Check sheet for the modelled part. Datum: model origin and axes. Units: mm. A direction names the side the tool comes from. Give positions to 0.01 mm unless a question says otherwise; leave off trailing zeros. Loops run counter-clockwise (first coordinate to the right, second up) from the corner with the lowest first, then second, coordinate; pieces in that order, holes last. Notation, with made-up numbers: M 5,28.5 L 58,28.5 A27 ccw 58,44.5 Z; hole C 4,82.25 d11. An arc over 180 degrees is marked long. Write each question's results on one line, items separated by ' | '. Start each with the question number.
1. Sectioned sample at C-C on z = -40.5. Record the cut outline in (x, y), and give its area (3 significant figures).
2. Sectioned sample at A-A on y = 0.25. Record the cut outline in (x, z), and give its area (3 significant figures).
3. Material ranges on line 1 along Z through (x, y) = (0.5, 9.75); line 2 along X through (y, z) = (-0.25, -38.5); line 3 along Y through (x, z) = (12, -32), recorded low to high.
4. Tool access check on faces 1 (the flat face through (0, -3.492, -30)), 2 (the flat face through (-17.78, 0, -30)), 3 (the flat face through (17.78, 0, -30)), 4 (the flat face through (0, 3.492, -30)). Record the directions out of +Z, -Z, +X, -X, +Y, -Y that give a thin tool (end or side, any length) a straight path to the whole face; none if there is none.
5. Sectioned sample at D-D on y = -9.25. Record the cut outline in (x, z), and give its area (3 significant figures).
6. Sectioned sample at B-B on x = 15. Record the cut outline in (y, z), and give its area (3 significant figures).
7. Go/stop test with flat-tipped pins: pin 1 (5 mm diameter, centred on x = -8.5, z = -36, fed in from -Y); pin 2 (2 mm diameter, centred on x = -26, y = 11, fed in from -Z); pin 3 (1 mm diameter, centred on x = 3, z = -37, fed in from +Y). Record where each tip stops, or that it passes through.
```python
from build123d import *

# Parameters (mm, degrees)
SKETCH1_W           = 70.0024
SKETCH1_H           = 22.9616
BOSS_EXTRUDE1_DEPTH = 14.9098
SKETCH2_W           = 35.56
SKETCH2_H           = 6.985
BOSS_EXTRUDE2_DEPTH = 38.1


with BuildPart() as part:
    # Sketch1 → Boss-Extrude1 (new, symmetric)
    with BuildSketch(Plane(origin=(0, 0, 0), x_dir=(1, 0, 0), z_dir=(0, 1, 0))):
        Rectangle(SKETCH1_W, SKETCH1_H)
    extrude(amount=BOSS_EXTRUDE1_DEPTH, both=True)

    # Sketch2 → Boss-Extrude2 (add)
    with BuildSketch(Plane(origin=(0, 0, -11.4808), x_dir=(-1, 0, 0), z_dir=(0, 0, -1))):
        Rectangle(SKETCH2_W, SKETCH2_H)
    extrude(amount=BOSS_EXTRUDE2_DEPTH)


solid = part.part
```
Output values:
1) outline: M -17.78,-3.49 L 17.78,-3.49 L 17.78,3.49 L -17.78,3.49 Z | area: 248 mm2
2) outline: M -35,-11.48 L -17.78,-11.48 L -17.78,-49.58 L 17.78,-49.58 L 17.78,-11.48 L 35,-11.48 L 35,11.48 L -35,11.48 Z | area: 2,960 mm2
3) line 1: -11.48 to 11.48 | line 2: -17.78 to 17.78 | line 3: -3.49 to 3.49
4) face 1: -Z, +X, -X, -Y | face 2: -Z, -X, +Y, -Y | face 3: -Z, +X, +Y, -Y | face 4: -Z, +X, -X, +Y
5) outline: M -35,-11.48 L 35,-11.48 L 35,11.48 L -35,11.48 Z | area: 1,610 mm2
6) outline: M -14.91,-11.48 L -3.49,-11.48 L -3.49,-49.58 L 3.49,-49.58 L 3.49,-11.48 L 14.91,-11.48 L 14.91,11.48 L -14.91,11.48 Z | area: 951 mm2
7) pin 1: y = -3.49 | pin 2: z = -11.48 | pin 3: y = 3.49
